Verification items for the finished model (mm, model axes). A direction names the side the tool comes from. Coordinates: 2 decimals unless noted, no trailing zeros. Order: outer loops, then holes, each group sorted by start corner. A loop starts at its lowest first (then second) coordinate and runs counter-clockwise, first axis right, second up. Notation, with made-up numbers: (-40, 43) -> (-34, 43) arc R25 ccw to (-34, 63) -> close; hole circle Ø4 at (23, -20.75). An arc over 180 degrees is marked (long way). Answer as CSV lines item,"result".
```python
from build123d import *

# Parameters (mm, degrees)
F1_DEPTH = 22.86
F2_R     = 1.905
F3_DEPTH = 50.8
F4_W     = 89.154
F4_H     = 0.508
F5_DEPTH = 19.05


with BuildPart() as f1:
    # F0 (on Front) → F1 (new body)
    with BuildSketch(Plane.XZ):
        with BuildLine():
            Line((0, 19.05), (0, 0))
            Line((0, 0), (96.774, 0))
            Line((96.774, 0), (96.774, 19.05))
            Line((96.774, 19.05), (93.276378, 19.05))
            ThreePointArc((93.276378, 19.05), (83.439, 3.81), (73.601622, 19.05))
            Line((73.601622, 19.05), (69.908378, 19.05))
            ThreePointArc((69.908378, 19.05), (60.071, 3.81), (50.233622, 19.05))
            Line((50.233622, 19.05), (46.540378, 19.05))
            ThreePointArc((46.540378, 19.05), (36.703, 3.81), (26.865622, 19.05))
            Line((26.865622, 19.05), (23.172378, 19.05))
            ThreePointArc((23.172378, 19.05), (13.335, 3.81), (3.497622, 19.05))
            Line((3.497622, 19.05), (0, 19.05))
        make_face()
    extrude(amount=F1_DEPTH)

    # F2 (on face) → F3 (cut)
    with BuildSketch(Plane.XZ.offset(22.86)):
        with Locations((24.765, 3.81)):
            Circle(F2_R)
        with Locations((48.26, 3.81)):
            Circle(F2_R)
        with Locations((71.755, 3.81)):
            Circle(F2_R)
        with Locations((3.81, 3.81)):
            Circle(F2_R)
        with Locations((92.964, 3.81)):
            Circle(F2_R)
    extrude(amount=-F3_DEPTH, mode=Mode.SUBTRACT)

    # F4 (on face) → F5 (cut)
    with BuildSketch(Plane.XZ.offset(22.86)):
        with Locations((48.387, 0.254)):
            Rectangle(F4_W, F4_H)
    extrude(amount=-F5_DEPTH, mode=Mode.SUBTRACT)


solid = f1.part
```
Item 1: Depth check by flat-ended pin: pin 1 Ø9.5 at (x, y) = (50, -9) entering from -Z; pin 2 Ø12 at (x, y) = (35.5, -8) entering from +Z; pin 3 Ø8 at (x, y) = (60.5, -6) entering from +Z. Enter the tip coordinate at first touch or a pass-through.
Answer list:
pin 1,"z = 0.51"
pin 2,"z = 6.56"
pin 3,"z = 4.76"
Item 2: Section check A-A, the plane y = -19. Record the boundary of the cut face in (x, z) (3 decimals), plus the area to 3 significant figures.
Answer list:
outline,"(0, 0) -> (3.81, 0) -> (3.81, 0.508) -> (92.964, 0.508) -> (92.964, 0) -> (96.774, 0) -> (96.774, 19.05) -> (93.276, 19.05) arc R10.795 cw (long way) to (73.602, 19.05) -> (69.908, 19.05) arc R10.795 cw (long way) to (50.234, 19.05) -> (46.54, 19.05) arc R10.795 cw (long way) to (26.866, 19.05) -> (23.172, 19.05) arc R10.795 cw (long way) to (3.498, 19.05) -> (0, 19.05) -> close; hole circle Ø3.81 at (3.81, 3.81); hole circle Ø3.81 at (24.765, 3.81); hole circle Ø3.81 at (48.26, 3.81); hole circle Ø3.81 at (71.755, 3.81); hole circle Ø3.81 at (92.964, 3.81)"
area,"636 mm2"
Item 3: Thickness scan on line 1 (X direction, y = -16.25, z = 10.5); line 2 (X direction, y = -11.75, z = 6.75); line 3 (Z direction, x = 5, y = -8.75). Record the ranges inside material, lowest first.
Answer list:
line 1,"0 to 3.35, 23.32 to 26.72, 46.69 to 50.09, 70.06 to 73.45, 93.42 to 96.77"
line 2,"0 to 5.93, 20.74 to 29.3, 44.11 to 52.67, 67.48 to 76.03, 90.84 to 96.77"
line 3,"0.51 to 2.32, 5.3 to 7.74"
Item 4: Section check D-D, the plane x = 37. Record the boundary of the cut face in (y, z), plus the area to 3 significant figures.
Answer list:
outline,"(-22.86, 0.51) -> (-3.81, 0.51) -> (-3.81, 0) -> (0, 0) -> (0, 3.81) -> (-22.86, 3.81) -> close"
area,"77.5 mm2"
Item 5: Section check C-C, the plane z = 3. Record the boundary of the cut face in (x, y).
Answer list:
outline,"(0, -22.86) -> (2.09, -22.86) -> (2.09, 0) -> (0, 0) -> close; (5.53, -22.86) -> (23.04, -22.86) -> (23.04, 0) -> (5.53, 0) -> close; (26.49, -22.86) -> (46.54, -22.86) -> (46.54, 0) -> (26.49, 0) -> close; (49.98, -22.86) -> (70.03, -22.86) -> (70.03, 0) -> (49.98, 0) -> close; (73.48, -22.86) -> (91.24, -22.86) -> (91.24, 0) -> (73.48, 0) -> close; (94.69, -22.86) -> (96.77, -22.86) -> (96.77, 0) -> (94.69, 0) -> close"
Item 6: Release check for a two-part mould opening along X. For faces 1 (the flat face through (72, -11, 19.05)), 2 (the cylindrical face through (83.74, -11.27, 3.814)), 3 (the cylindrical face through (13.636, -11.27, 3.814)), 4 (the flat face through (0, -11, 10)) record: +X half, -X half, draft (parallel to the pull), parting line (faces both ways), or undercut.
Answer list:
face 1,"draft"
face 2,"undercut"
face 3,"undercut"
face 4,"-X half"
Item 7: Tool access check on faces 5 (the flat face through (48, -13, 0.508)), 6 (the flat face through (96.774, -11, 9)). Record the directions out of +Z, -Z, +X, -X, +Y, -Y that give a thin tool (end or side, any length) a straight path to the whole face; none if there is none.
Answer list:
face 5,"-Z, -Y"
face 6,"+Z, -Z, +X, +Y, -Y"
Item 8: Section check B-B, the plane z = 8.25. Record the boundary of the cut face in (x, y), plus the area to 3 significant figures.
Answer list:
outline,"(0, -22.86) -> (4.61, -22.86) -> (4.61, 0) -> (0, 0) -> close; (22.06, -22.86) -> (27.98, -22.86) -> (27.98, 0) -> (22.06, 0) -> close; (45.43, -22.86) -> (51.34, -22.86) -> (51.34, 0) -> (45.43, 0) -> close; (68.8, -22.86) -> (74.71, -22.86) -> (74.71, 0) -> (68.8, 0) -> close; (92.17, -22.86) -> (96.77, -22.86) -> (96.77, 0) -> (92.17, 0) -> close"
area,"616 mm2"
